Print and shaded views of the part. All mm, measured from the part's lowest x, y and z. Coordinates: 2 decimals unless noted, no trailing zeros. Order: outer loops, then holes, each group sorted by start corner. A loop starts at its lowest first (then second) coordinate and runs counter-clockwise, first axis right, second up. Notation, with made-up numbers: M 23.25,6.5 L 39.25,6.5 A18 cw 39.25,30.5 Z; hole C -33.75,71.5 d1. An arc over 180 degrees is marked long. Use a Markdown table: item, result. Add a question column.
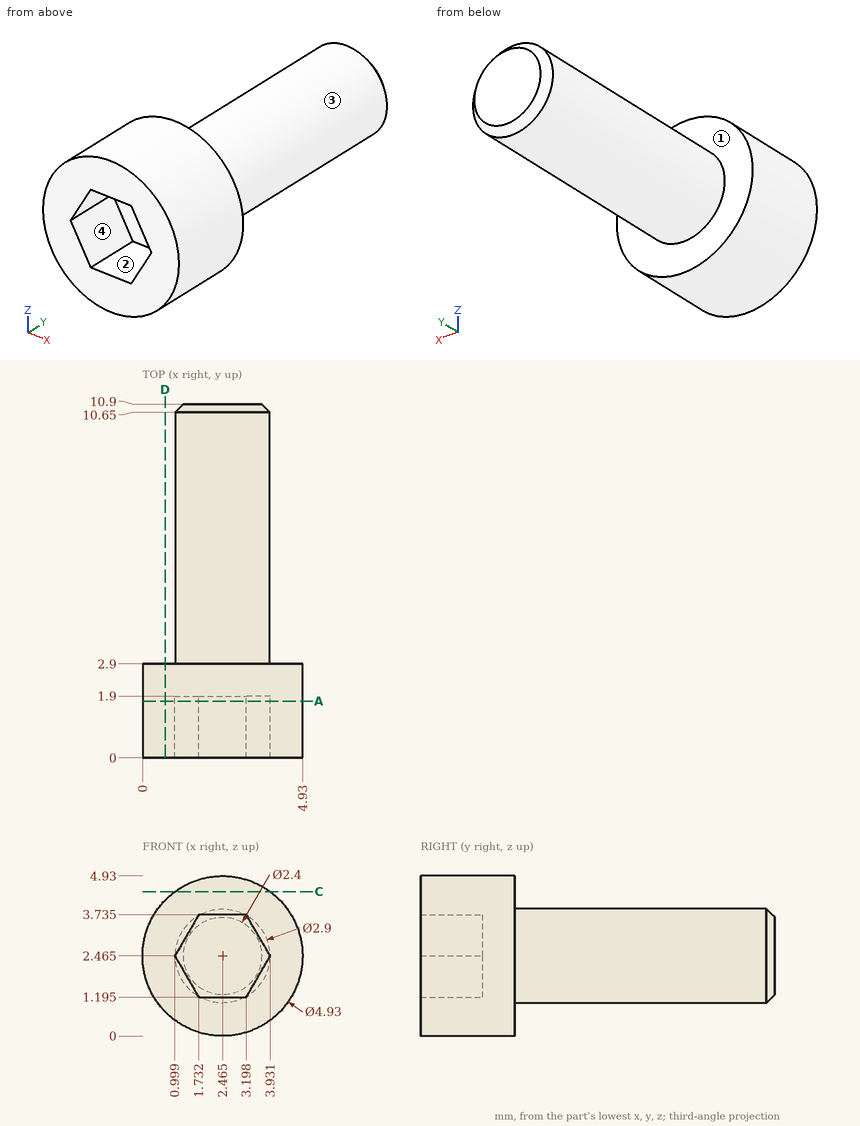
(1) Slice it at A-A on y = 1.75. Give the cut face in (x, z) (1 decimal), and give its area (3 significant figures).
(2) Drop flat-ended pins along their axis: P1, Ø1.5, axis at x = 4, y = 9.5, coming from the +Z side (1 decimal); P2, Ø1, axis at x = 1.5, y = 9.5, coming from the -Z side. Give the stop position or say it passes through.
(3) Slice it at D-D on x = 0.7. Give the cut face in (y, z) (1 decimal).
(4) Mould opens along X. For the marked faces 1, 2, 3 and 4 say: released by +X, released by -X, zero draft, split by the parting line, or undercut.
(5) Drill centre lines: line 1 along Y through (x, z) = (1.65, 4.35); line 2 along Y through (x, z) = (3.1, 2); line 3 along Z through (x, y) = (3.45, 3.5). Where is each one in solid material? Low to high. Write a range as from..to.
(6) Slice it at C-C on z = 4.45. Give the cut face in (x, y).
Solutions:
| question | item | result |
|---|---|---|
| 1 | outline | C 2.5,2.5 d4.9; hole M 1,2.5 L 1.7,1.2 L 3.2,1.2 L 3.9,2.5 L 3.2,3.7 L 1.7,3.7 Z |
| 1 | area | 13.5 mm² |
| 2 | P1 | z = 3.7 |
| 2 | P2 | z = 1.09 |
| 3 | outline | M 0,0.7 L 2.9,0.7 L 2.9,4.2 L 0,4.2 Z |
| 4 | face 1 | zero draft |
| 4 | face 2 | undercut |
| 4 | face 3 | split by the parting line |
| 4 | face 4 | undercut |
| 5 | line 1 | 0..2.9 |
| 5 | line 2 | 1.9..10.9 |
| 5 | line 3 | 1.4..3.53 |
| 6 | outline | M 1,0 L 3.93,0 L 3.93,2.9 L 1,2.9 Z |
